CAD build for the part. Positions are in the model's coordinates, mm. Give positions to 0.01 mm unless a question says otherwise; leave off trailing zeros. Write each loop counter-clockwise with the first axis right and the second up, starting at its lowest first coordinate (ties: lowest second). Pieces come first, ordered by that corner, then holes. Notation, with made-up numbers: (51.5, 50.25) - (92.5, 50.25) arc R24 ccw to (92.5, 77.25) - close; hole circle Ø10 at (-8.75, 45.5). An arc over 180 degrees is marked (long way). Put each result on its own line as item: value. Start each with the question number.
1. Cut at C-C on x = 38.5. List the corners of the cut face in (y, z), and give its area (3 significant figures).
2. Wall check: line 1 (X direction, y = 1.25, z = -66); line 2 (Z direction, x = -32, y = 4.75); line 3 (Z direction, x = 16.5, y = 2). Give the ranges that are in metal, low to high.
3. Cut at A-A on y = 2. Give the number of separate pieces and of enclosed holes in the cut face, and give its area (3 significant figures).
4. Cut at B-B on z = 23. List the corners of the cut face in (x, y), and give its area (3 significant figures).
5. Drop a flat-ended pin along its axis: pin 1 (3 mm diameter, centred on y = 4.5, z = -8.5, fed in from -X). Give the stop position or say it passes through.
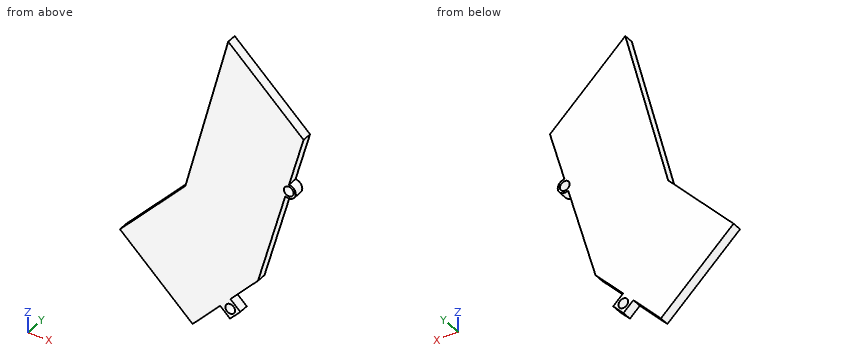
from build123d import *

# Parameters (mm, degrees)
SKETCH1_R           = 3.175
BOSS_EXTRUDE1_DEPTH = 6.35


with BuildPart() as part:
    # Sketch1 → Boss-Extrude1 (new body)
    with BuildSketch(Plane(origin=(0, 0, 0), x_dir=(1, 0, 0), z_dir=(0, 1, 0))):
        with BuildLine():
            Line((59.992329175, -52.562440303), (50.525242276, -18.985043707))
            ThreePointArc((50.525242276, -18.985043707), (54.736759655, -13.141199939), (48.092868173, -10.358019279))
            Line((48.092868173, -10.358019279), (30.218426447, 53.0381685))
            Line((30.218426447, 53.0381685), (12.190853288, 72.285391563))
            Line((12.190853288, 72.285391563), (18.653548719, 78.338561638))
            Line((18.653548719, 78.338561638), (11.968839999, 85.475522266))
            Line((11.968839999, 85.475522266), (5.506144568, 79.422352191))
            Line((5.506144568, 79.422352191), (-12.521428591, 98.669575253))
            Line((-12.521428591, 98.669575253), (-59.992329175, 54.206790652))
            Line((-59.992329175, 54.206790652), (-17.252470825, 8.575380364))
            Line((-17.252470825, 8.575380364), (10.765830225, -98.669575253))
            Line((10.765830225, -98.669575253), (59.992329175, -52.562440303))
        make_face()
        with Locations(Location((12.079948167, 78.880545368, 0), (0, 0, 270))):
            Circle(SKETCH1_R, mode=Mode.SUBTRACT)
        with Locations(Location((50.308887465, -14.389630582, 0), (0, 0, 270))):
            Circle(SKETCH1_R, mode=Mode.SUBTRACT)
    extrude(amount=BOSS_EXTRUDE1_DEPTH)


solid = part.part
Report:
1. outline: (0, -23.67) - (6.35, -23.67) - (6.35, 72.69) - (0, 72.69) - close
1. area: 612 mm²
2. line 1: x = -47.4 to 18.08
2. line 2: z = -80.43 to -24.32
2. line 3: z = -80.64 to -76.32, -67.68 to 93.3
3. separate pieces: 1
3. enclosed holes: 2
3. area: 10,600 mm²
4. outline: (-9, 0) - (51.66, 0) - (51.66, 6.35) - (-9, 6.35) - close
4. area: 385 mm²
5. pin 1: stops at x = -18.59
